from build123d import *

# Parameters (mm, degrees)
F2_DEPTH = 20
F3_R     = 5
F4_R     = 1
F6_START = -2.5
F6_DEPTH = 7.5
F7_R     = 2
F8_DEPTH = 25
F9_SIZE  = 1
F10_SIZE = 1


# Not quite as in the source:
# - a feature names something its author has since deleted; it is built from what else it names


with BuildPart() as f2:
    # F1 (on Top) → F2 (new body)
    with BuildSketch(Plane.XY):
        Polygon((0.75, 14.5), (-8, 14.5), (-8, -16), (16.5, -16), (16.5, 14.5), (7.75, 14.5), (7.75, 11.5), (9.5, 10.4896370289), (9.5, -10), (-1, -10), (-1, 10.4896370289), (0.75, 11.5), align=None)
    extrude(amount=F2_DEPTH)

    # F3
    f3_edges = [f2.edges().sort_by_distance(p)[0] for p in [
        (-8, 14.5, 10),
        (16.5, 14.5, 10),
        (-8, -16, 10),
        (16.5, -16, 10),
    ]]
    fillet(f3_edges, radius=F3_R)

    # F4
    f4_edges = [f2.edges().sort_by_distance(p)[0] for p in [
        (0.75, 11.5, 10),
        (7.75, 11.5, 10),
        (-1, 10.489637, 10),
        (9.5, 10.489637, 10),
        (9.5, -10, 10),
        (-1, -10, 10),
    ]]
    fillet(f4_edges, radius=F4_R)

    # F5 (on face) → F6 (cut)
    with BuildSketch(Plane.YZ.offset(-1).offset(F6_START)):
        Polygon((-7.897114317, 7.75), (-4, 5.5), (-0.102885683, 7.75), (-0.102885683, 12.25), (-4, 14.5), (-7.897114317, 12.25), align=None)
    extrude(amount=-F6_DEPTH, mode=Mode.SUBTRACT)

    # F7 (on face) → F8 (cut)
    with BuildSketch(Plane(origin=(-3.5, 0, 0), x_dir=(0, -1, 0), z_dir=(-1, 0, 0))):
        with Locations((4, 10)):
            Circle(F7_R)
    extrude(amount=-F8_DEPTH, mode=Mode.SUBTRACT)

    # F9
    f9_edges = [f2.edges().sort_by_distance(p)[0] for p in [
        (-8, -7.897114, 10),
        (-8, -5.948557, 13.375),
        (-8, -2.051443, 13.375),
        (-8, -0.102886, 10),
        (-8, -5.948557, 6.625),
        (-8, -2.051443, 6.625),
    ]]
    chamfer(f9_edges, length=F9_SIZE)

    # F10
    f10_edges = [f2.edges().sort_by_distance(p)[0] for p in [
        (16.5, -2, 10),
        (-1, -2, 10),
        (9.5, -2, 10),
    ]]
    chamfer(f10_edges, length=F10_SIZE)


solid = f2.part
Here's how the part is built. I have some questions about the finished solid (model axes, mm). A direction names the side the tool comes from. Round coordinates to 2 decimals unless told otherwise and drop trailing zeros. Write each loop counter-clockwise with the first axis right and the second up, starting at its lowest first coordinate (ties: lowest second). Pieces come first, ordered by that corner, then holes.
1. If we mould it in two halves opening along Y, with no side actions, what happens to faces 5 (the flat face through (10, 14.5, 10)), 6 (the flat face through (7.75, 13, 10)), 7 (the flat face through (-5.226, -5.976, 6.641))? For each: released by +Y, released by -Y, zero draft, split by the parting line, or undercut.
2. Suppose I cut it at A-A (z = 1.5). List the corners of the cut face in (x, y) for me.
3. For faces 1 (the cylindrical face through (7.89, 11.57, 10.14)), 2 (the flat face through (-5.23, -2.08, 6.61)), 3 (the flat face through (10, -1, 0)), 4 (the flat face through (0.75, 13, 10)), which set-ups out of +Z, -Z, +X, -X, +Y, -Y let a thin tool reach every point of the face, with its end or its side?
4. Suppose I cut it at B-B (x = -4.5). List the corners of the cut face in (y, z) for me.
5. Suppose I cut it at C-C (z = 10). State how many separate pieces and enclosed holes the cut face has, and give its area (3 significant figures).
6. Will these pins go through, and if not, where does the flat tip stop? pin 1 Ø4 at (y, z) = (-4, 12) entering from -X; pin 2 Ø3.5 at (y, z) = (-4, 10) entering from +X; pin 3 Ø4 at (x, z) = (3, 13.5) entering from +Y; pin 4 Ø5.5 at (y, z) = (-3.5, 8.5) entering from -X.
7. I need wall thicknesses on L1, parallel to X at y = 5, z = 4; L2, parallel to Z at x = 14.4, y = -4; L3, parallel to X at y = 11, z = 2. Which ranges of each line are inside material? Lowest first, please.
Answer sheet:
1. face 5: released by +Y
1. face 6: zero draft
1. face 7: undercut
2. outline: (-8, -11) arc R5 ccw to (-3, -16) - (11.5, -16) arc R5 ccw to (16.5, -11) - (16.5, 9.5) arc R5 ccw to (11.5, 14.5) - (7.75, 14.5) - (7.75, 12.08) arc R1 ccw to (8.25, 11.21) - (9, 10.78) arc R1 cw to (9.5, 9.91) - (9.5, -9) arc R1 cw to (8.5, -10) - (0, -10) arc R1 cw to (-1, -9) - (-1, 9.91) arc R1 cw to (-0.5, 10.78) - (0.25, 11.21) arc R1 ccw to (0.75, 12.08) - (0.75, 14.5) - (-3, 14.5) arc R5 ccw to (-8, 9.5) - close
3. face 1: +Z, -Z
3. face 2: -X
3. face 3: -Z, +X, -X, +Y, -Y
3. face 4: +Z, -Z, +Y
4. outline: (-15.77, 0) - (14.27, 0) - (14.27, 20) - (-15.77, 20) - close; hole (-7.9, 7.75) - (-4, 5.5) - (-0.1, 7.75) - (-0.1, 12.25) - (-4, 14.5) - (-7.9, 12.25) - close
5. separate pieces: 3
5. enclosed holes: 0
5. area: 404 mm2
6. pin 1: stops at x = -3.5
6. pin 2: passes through
6. pin 3: stops at y = -10
6. pin 4: stops at x = -7.4
7. L1: x = -8 to -1, 9.5 to 16.5
7. L2: z = 0 to 8, 12 to 20
7. L3: x = -7.77 to -0.12, 8.62 to 16.27
